Check sheet for the drawn part. Datum: minimum x, y, z corner. Units: mm. A direction names the side the tool comes from. Coordinates: 2 decimals unless noted, no trailing zeros. Write each loop counter-clockwise with the first axis right and the second up, starting at its lowest first coordinate (ties: lowest second). Pieces come first, ordered by that corner, then holes. Notation, with made-up numbers: (-12, 1.5) -> (22, 1.5) arc R24 cw to (22, 36.5) -> close; hole circle Ø10 at (68.25, -29). An arc over 180 degrees is marked (long way). Answer in a Markdown table with one row per item.
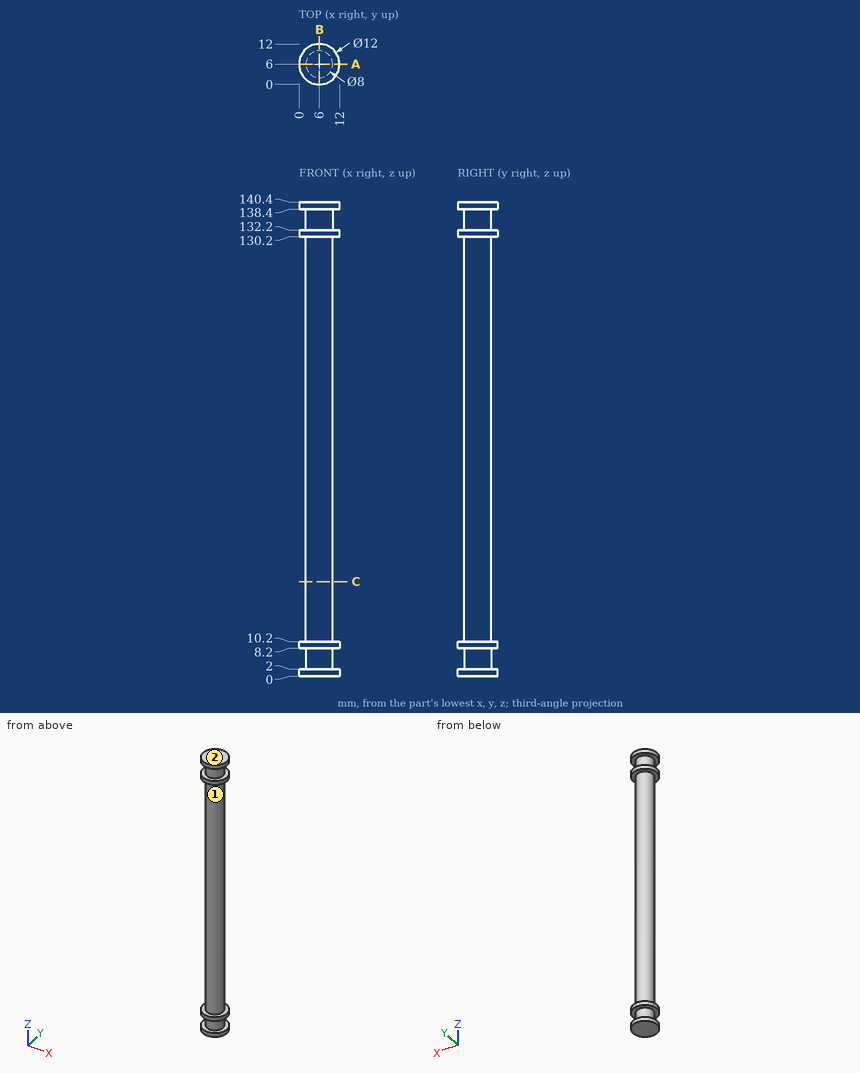
1. Material ranges on probe 1 along Z at (x, y) = (9.75, 4.25); probe 2 along Y at (x, z) = (5.75, 104); probe 3 along Y at (x, z) = (3.5, 74.5), recorded low to high. Write a range as from..to.
Findings below:
| item | result |
|---|---|
| probe 1 | z = 0..2, 8.2..10.2, 130.2..132.2, 138.4..140.4 |
| probe 2 | y = 2.01..9.99 |
| probe 3 | y = 2.88..9.12 |
2. Go/stop test with flat-tipped pins: pin 1 (1 mm diameter, centred on x = 8, z = 105, fed in from -Y); pin 2 (1 mm diameter, centred on y = 8.5, z = 54, fed in from +X); pin 3 (3.5 mm diameter, centred on x = 3.5, y = 6, fed in from -Z); pin 4 (4 mm diameter, centred on y = 11, z = 66.5, fed in from +X). Record where each tip stops, or that it passes through.
Findings below:
| item | result |
|---|---|
| pin 1 | stops at y = 2.29 |
| pin 2 | stops at x = 9.46 |
| pin 3 | stops at z = 0 |
| pin 4 | stops at x = 8.65 |
3. Sectioned sample at C-C, the plane z = 28. Record the cut outline in (x, y).
Findings below:
| item | result |
|---|---|
| outline | circle Ø8 at (6, 6) |
4. Sectioned sample at A-A, the plane y = 6. Record the cut outline in (x, z), and give its area (3 significant figures).
Findings below:
| item | result |
|---|---|
| outline | (0, 0) -> (12, 0) -> (12, 2) -> (10, 2) -> (10, 8.2) -> (12, 8.2) -> (12, 10.2) -> (10, 10.2) -> (10, 130.2) -> (12, 130.2) -> (12, 132.2) -> (10, 132.2) -> (10, 138.4) -> (12, 138.4) -> (12, 140.4) -> (0, 140.4) -> (0, 138.4) -> (2, 138.4) -> (2, 132.2) -> (0, 132.2) -> (0, 130.2) -> (2, 130.2) -> (2, 10.2) -> (0, 10.2) -> (0, 8.2) -> (2, 8.2) -> (2, 2) -> (0, 2) -> close |
| area | 1,160 mm² |
5. Access from +Z, -Z, +X, -X, +Y, -Y to the whole of each face (thin tool, end or side, straight path). Record for the marked faces 1 and 2.
Findings below:
| item | result |
|---|---|
| face 1 | none |
| face 2 | +Z, +X, -X, +Y, -Y |
